Check sheet for the drawn part. Datum: minimum x, y, z corner. Units: mm. A direction names the side the tool comes from. Round coordinates to 2 decimals unless told otherwise and drop trailing zeros. Loops run counter-clockwise (first coordinate to the right, second up) from the corner with the lowest first, then second, coordinate; pieces in that order, holes last.
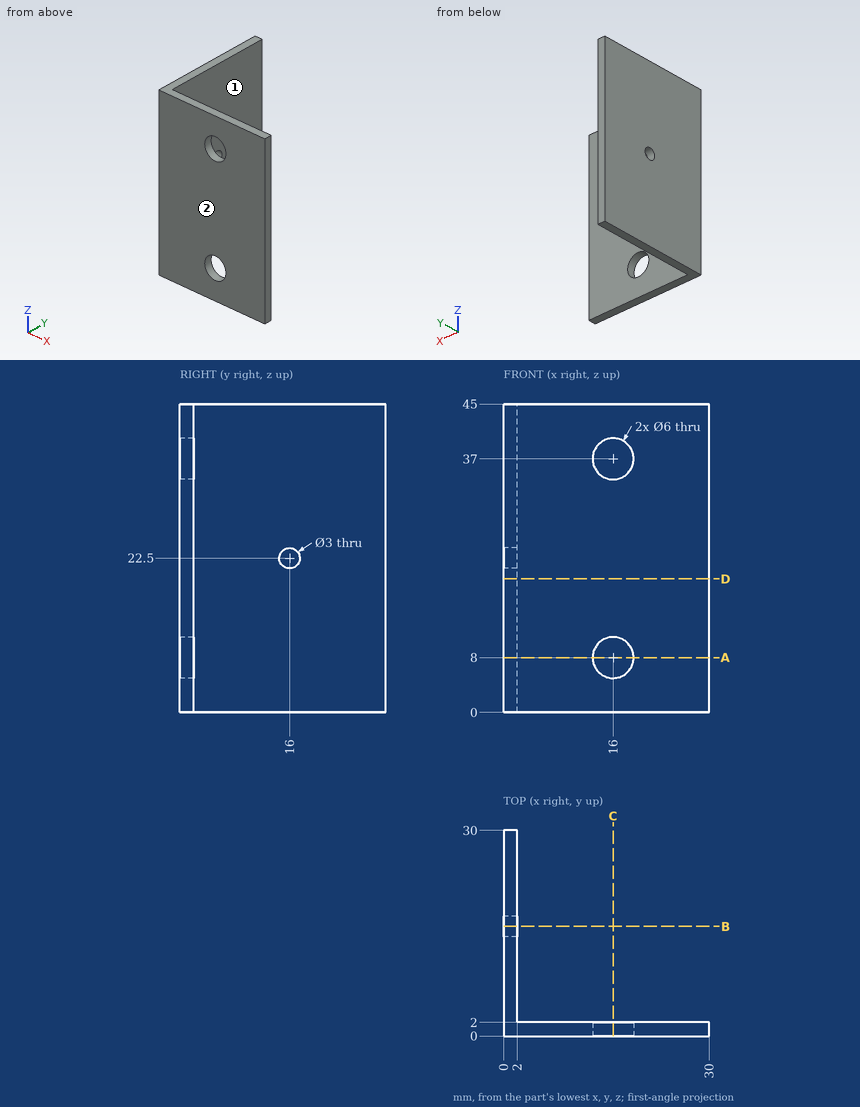
1) Scan lines: line 1 along Y through (x, z) = (0.7, 22.5); line 2 along Y through (x, z) = (21.5, 8). Record each from-to range of solid material in increasing order.
Report:
line 1: y = 0 to 14.5, 17.5 to 30
line 2: y = 0 to 2
2) Access from +Z, -Z, +X, -X, +Y, -Y to the whole of each face (thin tool, end or side, straight path). Record for the marked faces 1 and 2.
Report:
face 1: +Z, -Z, +X, +Y
face 2: +Z, -Z, +X, -X, -Y
3) Sectioned sample at D-D, the plane z = 19.5. Record the cut outline in (x, y), then the cut area to 3 significant figures.
Report:
outline: (0, 0) - (30, 0) - (30, 2) - (2, 2) - (2, 30) - (0, 30) - close
area: 116 mm2
4) Gauge pin test, flat ends, axial feed: pin 1 (14 mm diameter, centred on x = 10.5, z = 12.5, fed in from +Y); pin 2 (1.5 mm diameter, centred on y = 8, z = 17, fed in from +X). Record the tip position at first contact, or that the pin passes through.
Report:
pin 1: stops at y = 2
pin 2: stops at x = 2
5) Sectioned sample at C-C, the plane x = 16. Record the cut outline in (y, z).
Report:
outline: (0, 0) - (2, 0) - (2, 5) - (0, 5) - close; (0, 11) - (2, 11) - (2, 34) - (0, 34) - close; (0, 40) - (2, 40) - (2, 45) - (0, 45) - close
6) Sectioned sample at A-A, the plane z = 8. Record the cut outline in (x, y).
Report:
outline: (0, 0) - (13, 0) - (13, 2) - (2, 2) - (2, 30) - (0, 30) - close; (19, 0) - (30, 0) - (30, 2) - (19, 2) - close
7) Sectioned sample at B-B, the plane y = 16. Record the cut outline in (x, z), then the cut area to 3 significant figures.
Report:
outline: (0, 0) - (2, 0) - (2, 21) - (0, 21) - close; (0, 24) - (2, 24) - (2, 45) - (0, 45) - close
area: 84.0 mm2
